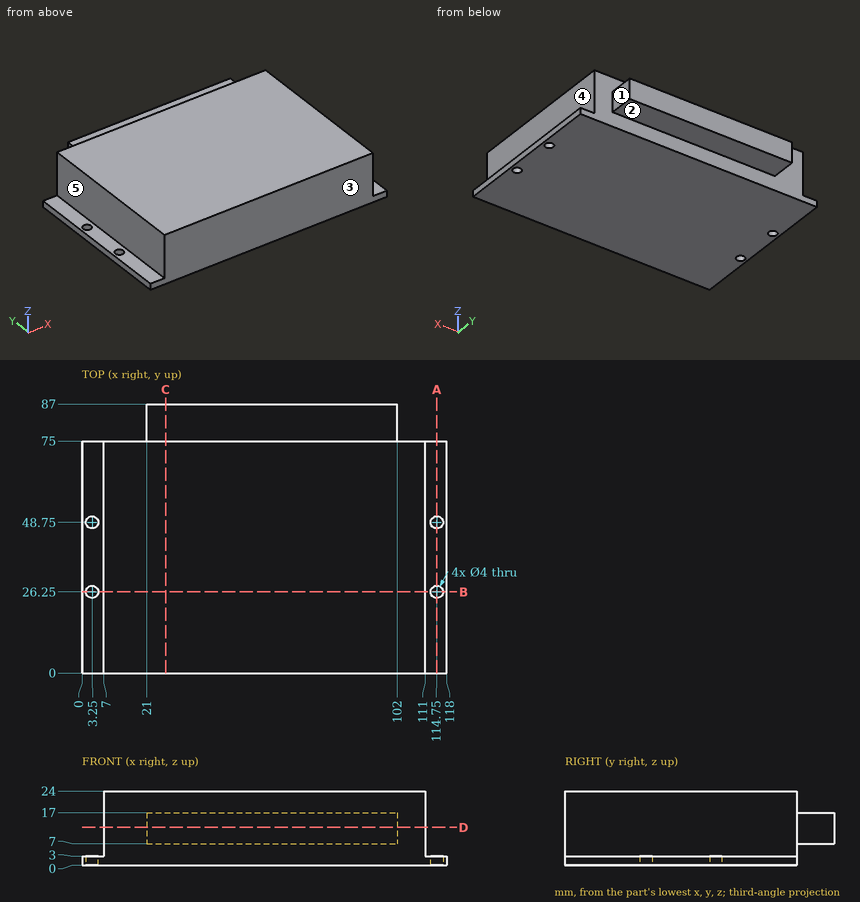
Input: dimensioned drawing with shaded views. Units: mm. Origin: part minimum x, y, z. A direction names the side the tool comes from. Give positions to 0.01 mm unless a question says otherwise; leave off trailing zeros. Loops run counter-clockwise (first coordinate to the right, second up) from the corner with the lowest first, then second, coordinate; pieces in that order, holes last. Notation, with made-up numbers: (54.25, -27.75) -> (68.25, -27.75) arc R33 ccw to (68.25, 9.25) -> close; hole circle Ø8 at (7.5, 37). An arc over 180 degrees is marked (long way). Use a Markdown table: item, result.
Q1. Access query for the marked faces 1, 2, 3, 4 and 5. Directions: +Z, -Z, +X, -X, +Y, -Y. A direction counts if a zero-diameter tool reaches every point of the face in a straight line with its end or side. Return the directions, or none.
Entries:
| item | result |
|---|---|
| face 1 | +Z, -Z, +X, +Y |
| face 2 | -Z, +X, -X, +Y |
| face 3 | +Z, -Z, +X, -X, -Y |
| face 4 | +Z, +X, +Y, -Y |
| face 5 | +Z, -X, +Y, -Y |
Q2. Ray query, probe 1 along Y at (x, z) = (3.25, 1.55); probe 2 along X at (y, z) = (60, 21.25); probe 3 along Y at (x, z) = (64, 18.5). Return the intervals inside material, ascending. Write a range as from..to.
Entries:
| item | result |
|---|---|
| probe 1 | y = 0..24.25, 28.25..46.75, 50.75..75 |
| probe 2 | x = 7..111 |
| probe 3 | y = 0..75 |
Q3. Section query A-A, the plane x = 114.75. Return the cut outline in (y, z), plus the area to 3 significant figures.
Entries:
| item | result |
|---|---|
| outline | (0, 0) -> (24.25, 0) -> (24.25, 3) -> (0, 3) -> close; (28.25, 0) -> (46.75, 0) -> (46.75, 3) -> (28.25, 3) -> close; (50.75, 0) -> (75, 0) -> (75, 3) -> (50.75, 3) -> close |
| area | 201 mm² |
Q4. Section query D-D, the plane z = 12.25. Return the cut outline in (x, y).
Entries:
| item | result |
|---|---|
| outline | (7, 0) -> (111, 0) -> (111, 75) -> (102, 75) -> (102, 87) -> (21, 87) -> (21, 75) -> (7, 75) -> close |
Q5. Section query B-B, the plane y = 26.25. Return the cut outline in (x, z), plus the area to 3 significant figures.
Entries:
| item | result |
|---|---|
| outline | (0, 0) -> (1.25, 0) -> (1.25, 3) -> (0, 3) -> close; (5.25, 0) -> (112.75, 0) -> (112.75, 3) -> (111, 3) -> (111, 24) -> (7, 24) -> (7, 3) -> (5.25, 3) -> close; (116.75, 0) -> (118, 0) -> (118, 3) -> (116.75, 3) -> close |
| area | 2,510 mm² |
Q6. First-contact query: P1, Ø9.5, axis at x = 80, y = 80.5, coming from the -Z side; P2, Ø8, axis at y = 45, z = 3.5, coming from the -X side; P3, Ø3, axis at x = 114.75, y = 48.75, coming from the +Z side; P4, Ø2, axis at y = 73, z = 6, coming from the +X side. Flat tips, straight axial feed; report the tip coordinate or a pass-through.
Entries:
| item | result |
|---|---|
| P1 | stops at z = 7 |
| P2 | stops at x = 0 |
| P3 | passes through |
| P4 | stops at x = 111 |
Q7. Section query C-C, the plane x = 27. Return the cut outline in (y, z).
Entries:
| item | result |
|---|---|
| outline | (0, 0) -> (75, 0) -> (75, 7) -> (87, 7) -> (87, 17) -> (75, 17) -> (75, 24) -> (0, 24) -> close |
